Design review of the part built by this model. Coordinates are the model's own, in mm. Round coordinates to 2 decimals unless told otherwise and drop trailing zeros. Order: outer loops, then holes, each group sorted by start corner. A loop starts at its lowest first (then second) coordinate and runs counter-clockwise, first axis right, second up. Notation, with made-up numbers: M 7.25,3.5 L 38.25,3.5 A25 ccw 38.25,23.5 Z; hole C 59.25,42 d8. An arc over 180 degrees is marked long. Write each question's results on one line, items separated by ' | '. Start each with the question number.
Item 1: Clearance check with flat-ended pins moving along their axes: pin 1 (3 mm diameter, centred on x = 70, z = 4, fed in from -Y); pin 2 (2 mm diameter, centred on x = -17.5, z = 2.5, fed in from +Y); pin 3 (15.5 mm diameter, centred on x = -84.85, y = -84.85, fed in from +Z); pin 4 (1 mm diameter, centred on y = -74, z = 6, fed in from -X). State where each tip first meets the part, or that it passes through.
Item 2: Take a section at B-B, the plane x = -17. Write out the cut boundary in (y, z), plus the area to 3 significant figures.
Item 3: The part is to be moulded in two halves that separate along Y. For faces 1 (the flat face through (61, -61, 8)), 2 (the cylindrical face through (-2.55, -111.89, 4.06)), 3 (the cylindrical face through (-105.028, -96.308, 3.944)), 4 (the cylindrical face through (-111.89, 2.55, 4.06)), say which applies: +Y half, -Y half, draft (parallel to the pull), parting line (faces both ways), or undercut.
Item 4: Wall thickness on line 1 (X direction, y = -91, z = 7.5); line 2 (Y direction, x = -2.5, z = 5.25); line 3 (Y direction, x = 18.5, z = 3): over which ranges is each line inside the solid? List them lowest first. Write a range as [from, to].
Item 5: Take a section at A-A, the plane y = 69.5. Write out the cut boundary in (x, z), plus the area to 3 significant figures.
Item 6: Take a section at C-C, the plane z = 5. Count the separate pieces of the cut face and the enclosed holes in it, plus the area to 3 significant figures.
Autodesk Inventor part; units mm, degrees
ref_plane "YZ Plane" through (0, 0, 0) normal (1, 0, 0) x (0, 1, 0)
ref_plane "XZ Plane" through (0, 0, 0) normal (0, 1, 0) x (-1, 0, 0)
ref_plane "XY Plane" through (0, 0, 0) normal (0, 0, 1) x (1, 0, 0)
sketch "Sketch2" plane through (0, 0, 0) normal (0, 0, 1) x (1, 0, 0)
  circle A0 centre (0, 0) radius 85
  circle A1 centre (0, 0) radius 142.5
  dimension "d25" = 170
  dimension "d27" = 285
extrude "Plate2" add sketch "Sketch2" along normal blind 8
sketch "Sketch3" plane through (0, 0, 8) normal (0, 0, 1) x (1, 0, 0)
  circle A0 centre (-120, 0) radius 8.5
  circle A1 centre (0, 0) radius 120 construction
  dimension "d28" = 240
  dimension "d15" = 17
extrude "Cut1" cut sketch "Sketch3" against normal blind 8
pattern_circular "Circular Pattern1" count 8 over 360 about axis through (0, 0, 0) along (0, 0, 1) of "Cut1"
equation "\"d17\" = Thickness"
equation "\"d14\" = Thickness"
equation "\"BendReliefWidth\" = Thickness"
equation "\"BendReliefDepth\" = 0.5 * Thickness"
equation "\"CornerReliefSize\" = 4 * Thickness"
equation "\"MinimumRemnant\" = 2 * Thickness"
equation "\"TransitionRadius\" = BendRadius"
equation "\"JacobiRadiusSize\" = BendRadius"
equation "\"GapSize\" = Thickness"
properties part number "PNS-733 charging flange round" material "Steel"
Results list:
1) pin 1: y = -124.96 | pin 2: y = 141.54 | pin 3: through | pin 4: x = -122.08
2) outline: M -141.48,0 L -83.28,0 L -83.28,8 L -141.48,8 Z; M 83.28,0 L 141.48,0 L 141.48,8 L 83.28,8 Z | area: 931 mm²
3) face 1: draft | face 2: undercut | face 3: parting line | face 4: undercut
4) line 1: [-109.66, -90.72], [-78.98, 78.98], [90.72, 109.66] | line 2: [-142.48, -128.12], [-111.88, -84.96], [84.96, 111.88], [128.12, 142.48] | line 3: [-141.29, -82.96], [82.96, 141.29]
5) outline: M -124.4,0 L -48.94,0 L -48.94,8 L -124.4,8 Z; M 48.94,0 L 124.4,0 L 124.4,8 L 48.94,8 Z | area: 1,210 mm²
6) separate pieces: 1 | enclosed holes: 9 | area: 39,300 mm²
